The listing builds one solid part. Answer for the finished solid, in the listing's coordinates (mm). Coordinates: 2 decimals unless noted, no trailing zeros. Order: outer loops, then holes, each group sorted by start corner. A loop starts at its lowest first (then second) coordinate and runs counter-clockwise, first axis right, second up. Notation, with made-up numbers: (57, 83.25) -> (74, 83.25) arc R30 cw to (74, 112.25) -> close; hole circle Ø5 at (58.25, 68.25). An arc over 180 degrees is marked (long way). Return JSON: item names as keys, results as strings.
```python
from build123d import *

# Parameters (mm, degrees)
ESQUISSE1_W                     = 355.6
ESQUISSE1_H                     = 368.3
BOSS_EXTRU_1_DEPTH              = 6.35
ESQUISSE2_W                     = 6.35
ESQUISSE2_H                     = 25.4
ENL_V_MAT_EXTRU_1_DEPTH         = 6.35
R_P_TITION_LIN_AIRE1_COUNT      = 7
R_P_TITION_LIN_AIRE1_PITCH      = 50.8
R_P_TITION_LIN_AIRE1_COUNT_DIR2 = 2
R_P_TITION_LIN_AIRE1_PITCH_DIR2 = 349.25
ESQUISSE3_W                     = 25.4
ESQUISSE3_H                     = 6.35
ENL_V_MAT_EXTRU_2_DEPTH         = 6.35
R_P_TITION_LIN_AIRE2_COUNT      = 7
R_P_TITION_LIN_AIRE2_PITCH      = 50.8
ESQUISSE4_W                     = 25.4
ESQUISSE4_H                     = 6.35
ENL_V_MAT_EXTRU_3_DEPTH         = 6.35
R_P_TITION_LIN_AIRE3_COUNT      = 7
R_P_TITION_LIN_AIRE3_PITCH      = 50.8
ESQUISSE5_W                     = 12.7
ESQUISSE5_H                     = 6.35
ENL_V_MAT_EXTRU_4_DEPTH         = 6.35
SKETCH3_W                       = 355.521495667
SKETCH3_H                       = 214.90407248
BOSS_EXTRUDE1_DEPTH             = 6.35
CUT_EXTRUDE2_DEPTH              = 331.396716197


with BuildPart() as part:
    # Esquisse1 → Boss.-Extru.1 (new body)
    with BuildSketch(Plane(origin=(0, 0, 0), x_dir=(1, 0, 0), z_dir=(0, 1, 0))):
        Rectangle(ESQUISSE1_W, ESQUISSE1_H)
    extrude(amount=BOSS_EXTRU_1_DEPTH)

    # Esquisse2 → Enlèv. mat.-Extru.1 (cut)
    with BuildSketch(Plane(origin=(0, 6.35, 0), x_dir=(1, 0, 0), z_dir=(0, 1, 0))):
        with Locations((174.625, -149.225)):
            Rectangle(ESQUISSE2_W, ESQUISSE2_H)
    enl_v_mat_extru_1 = extrude(amount=-ENL_V_MAT_EXTRU_1_DEPTH, mode=Mode.SUBTRACT)

    # Répétition linéaire1: Enl_v. mat.-Extru.1 7 × 2
    with Locations(*[(-j * R_P_TITION_LIN_AIRE1_PITCH_DIR2, 0, -i * R_P_TITION_LIN_AIRE1_PITCH) for i in range(R_P_TITION_LIN_AIRE1_COUNT) for j in range(R_P_TITION_LIN_AIRE1_COUNT_DIR2) if (i, j) != (0, 0)]):
        add(enl_v_mat_extru_1, mode=Mode.SUBTRACT)

    # Esquisse3 → Enlèv. mat.-Extru.2 (cut)
    with BuildSketch(Plane(origin=(0, 6.35, 0), x_dir=(1, 0, 0), z_dir=(0, 1, 0))):
        with Locations((-152.4, -180.975)):
            Rectangle(ESQUISSE3_W, ESQUISSE3_H)
    enl_v_mat_extru_2 = extrude(amount=-ENL_V_MAT_EXTRU_2_DEPTH, mode=Mode.SUBTRACT)

    # Répétition linéaire2: Enlèv. mat.-Extru.2 ×7
    with Locations(*[(i * R_P_TITION_LIN_AIRE2_PITCH, 0, 0) for i in range(1, R_P_TITION_LIN_AIRE2_COUNT)]):
        add(enl_v_mat_extru_2, mode=Mode.SUBTRACT)

    # Esquisse4 → Enlèv. mat.-Extru.3 (cut)
    with BuildSketch(Plane(origin=(0, 6.35, 0), x_dir=(1, 0, 0), z_dir=(0, 1, 0))):
        with Locations((-152.4, -60.325)):
            Rectangle(ESQUISSE4_W, ESQUISSE4_H)
    enl_v_mat_extru_3 = extrude(amount=-ENL_V_MAT_EXTRU_3_DEPTH, mode=Mode.SUBTRACT)

    # Répétition linéaire3: Enlèv. mat.-Extru.3 ×7
    with Locations(*[(i * R_P_TITION_LIN_AIRE3_PITCH, 0, 0) for i in range(1, R_P_TITION_LIN_AIRE3_COUNT)]):
        add(enl_v_mat_extru_3, mode=Mode.SUBTRACT)

    # Esquisse5 → Enlèv. mat.-Extru.4 (cut)
    with BuildSketch(Plane(origin=(0, 6.35, 0), x_dir=(1, 0, 0), z_dir=(0, 1, 0))):
        with Locations((-165.1, 180.975)):
            Rectangle(ESQUISSE5_W, ESQUISSE5_H)
        with Locations((165.1, 180.975)):
            Rectangle(ESQUISSE5_W, ESQUISSE5_H)
        with Locations((-139.7, 180.975)):
            Rectangle(ESQUISSE5_W, ESQUISSE5_H)
        with Locations((-114.3, 180.975)):
            Rectangle(ESQUISSE5_W, ESQUISSE5_H)
        with Locations((-88.9, 180.975)):
            Rectangle(ESQUISSE5_W, ESQUISSE5_H)
    extrude(amount=-ENL_V_MAT_EXTRU_4_DEPTH, mode=Mode.SUBTRACT)

    # Sketch3 → Boss-Extrude1 (add)
    with BuildSketch(Plane(origin=(0, 6.35, 0), x_dir=(1, 0, 0), z_dir=(0, 1, 0))):
        with Locations((-0.039252167, -170.95203624)):
            Rectangle(SKETCH3_W, SKETCH3_H)
    extrude(amount=-BOSS_EXTRUDE1_DEPTH)

    # Sketch1 → Cut-Extrude2 (cut, through all)
    with BuildSketch(Plane(origin=(0, 6.35, 0), x_dir=(1, 0, 0), z_dir=(0, 1, 0))):
        with BuildLine():
            Line((-95.25, -215.9), (95.25, -215.9))
            ThreePointArc((95.25, -215.9), (104.230256121, -212.180256121), (107.95, -203.2))
            Line((107.95, -203.2), (107.95, -63.5))
            Line((107.95, -63.5), (177.8, -63.5))
            Line((177.8, -63.5), (177.8, -278.40407248))
            Line((177.8, -278.40407248), (-177.8, -278.40407248))
            Line((-177.8, -278.40407248), (-177.8, -63.5))
            Line((-177.8, -63.5), (-107.95, -63.5))
            Line((-107.95, -63.5), (-107.95, -203.2))
            ThreePointArc((-107.95, -203.2), (-104.230256121, -212.180256121), (-95.25, -215.9))
        make_face()
    extrude(amount=-CUT_EXTRUDE2_DEPTH, mode=Mode.SUBTRACT)


solid = part.part
```
Item 1: The part is cut by section B-B on y = 4. Count the separate pieces of the cut face and the enclosed holes in it, plus the area to 3 significant figures.
Answer list:
{"separate pieces": "1", "enclosed holes": "3", "area": "118,000 mm2"}
Item 2: Flat-ended cylindrical pins translate along their axes: pin 1 (3 mm diameter, centred on y = 3, z = -159, fed in from +X); pin 2 (3 mm diameter, centred on x = -137.5, y = 2.5, fed in from -Z); pin 3 (1.9 mm diameter, centred on x = -175.5, y = 4, fed in from +Z). Find the tip coordinate at first contact, or state that the pin passes through.
Answer list:
{"pin 1": "x = 171.45", "pin 2": "z = -177.8", "pin 3": "z = 63.5"}
Item 3: The part is cut by section A-A on x = -57.5. Determine the outline of the cut face in (y, z), plus the area to 3 significant figures.
Answer list:
{"outline": "(0, -184.15) -> (6.35, -184.15) -> (6.35, 57.15) -> (0, 57.15) -> close; (0, 63.5) -> (6.35, 63.5) -> (6.35, 215.9) -> (0, 215.9) -> close", "area": "2,500 mm2"}
Item 4: The part is cut by section C-C on z = 137.5. Determine the outline of the cut face in (x, y), plus the area to 3 significant figures.
Answer list:
{"outline": "(-107.95, 0) -> (107.95, 0) -> (107.95, 6.35) -> (-107.95, 6.35) -> close", "area": "1,370 mm2"}
Item 5: Find the intervals of material crossed by probe 1 along Z at (x, y) = (61.5, 4.25); probe 2 along X at (y, z) = (1, 82); probe 3 along Z at (x, y) = (-161.5, 3), in increasing order.
Answer list:
{"probe 1": "-184.15 to 57.15, 63.5 to 215.9", "probe 2": "-107.95 to 107.95", "probe 3": "-177.8 to 57.15"}
